The figure shows three views and two pictorial views of one solid part (mm, origin at its lowest corner). Answer the questions. Coordinates: 2 decimals unless noted, no trailing zeros. Order: outer loops, then holes, each group sorted by start corner. A loop starts at its lowest first (then second) coordinate and runs counter-clockwise, first axis right, second up. Notation, with made-up numbers: (59.5, 84.25) -> (101.5, 84.25) arc R28 ccw to (101.5, 106.25) -> close; hole circle Ø11 at (-2, 31.5). An arc over 180 degrees is marked (long way). Use one line per item in the form item = value.
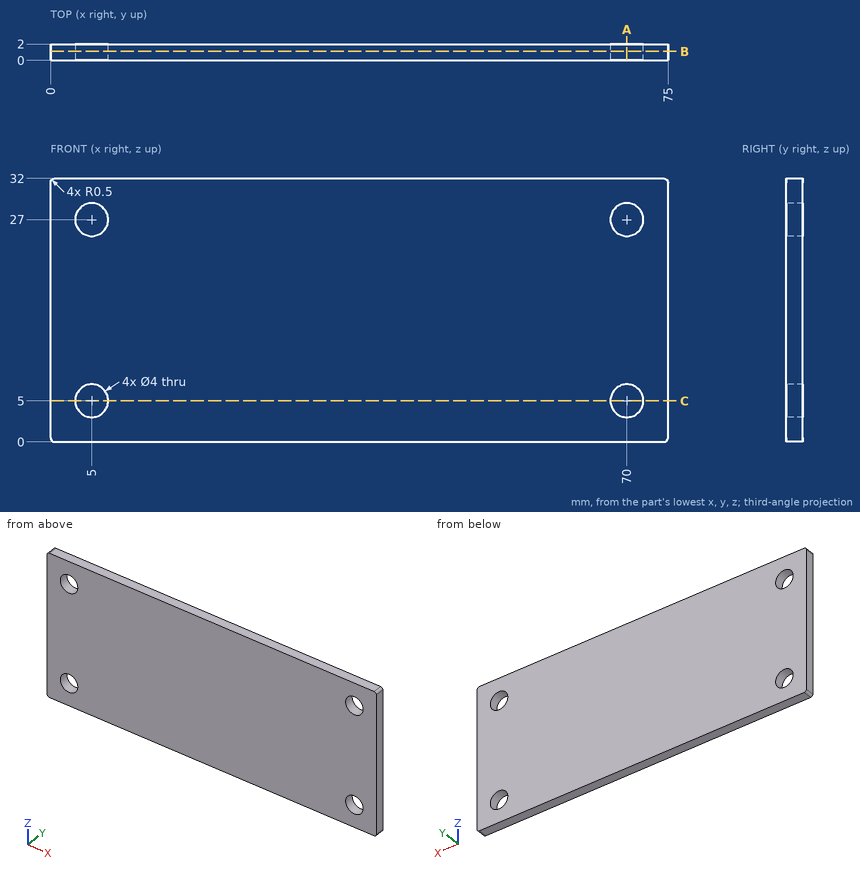
(1) Section A-A on x = 70 is taken. Write down the section's boundary in (y, z), plus the area to 3 significant figures.
Data:
outline = (0, 0) -> (2, 0) -> (2, 3) -> (0, 3) -> close; (0, 7) -> (2, 7) -> (2, 25) -> (0, 25) -> close; (0, 29) -> (2, 29) -> (2, 32) -> (0, 32) -> close
area = 48.0 mm²
(2) Straight lines are drawn through the part: line 1 along Z through (x, y) = (70, 1.3); line 2 along X through (y, z) = (0.25, 26.5). For each, find the intervals that lie inside material, in ascending order.
Data:
line_1 = 0 to 3, 7 to 25, 29 to 32
line_2 = 0 to 3.06, 6.94 to 68.06, 71.94 to 75
(3) Section B-B on y = 1.1 is taken. Write down the section's boundary in (x, z), plus the area to 3 significant figures.
Data:
outline = (0, 0.5) arc R0.5 ccw to (0.5, 0) -> (74.5, 0) arc R0.5 ccw to (75, 0.5) -> (75, 31.5) arc R0.5 ccw to (74.5, 32) -> (0.5, 32) arc R0.5 ccw to (0, 31.5) -> close; hole circle Ø4 at (5, 5); hole circle Ø4 at (5, 27); hole circle Ø4 at (70, 5); hole circle Ø4 at (70, 27)
area = 2,350 mm²
(4) Section C-C on z = 5 is taken. Write down the section's boundary in (x, y).
Data:
outline = (0, 0) -> (3, 0) -> (3, 2) -> (0, 2) -> close; (7, 0) -> (68, 0) -> (68, 2) -> (7, 2) -> close; (72, 0) -> (75, 0) -> (75, 2) -> (72, 2) -> close
